Verification items for the finished model (mm, model axes). Face numbers are marked on the shaded views. A direction names the side the tool comes from. Give positions to 0.01 mm unless a question says otherwise; leave off trailing zeros. Order: outer loops, then holes, each group sorted by start corner. A loop starts at its lowest first (then second) coordinate and runs counter-clockwise, first axis right, second up. Notation, with made-up numbers: M 49,24 L 79,24 A16 ccw 79,39 Z; hole C -30.75,65 d8. An arc over 180 degrees is marked long. Answer as a JSON object with one key per item and string values.
Autodesk Inventor part; units mm, degrees
ref_plane "YZ Plane" through (0, 0, 0) normal (1, 0, 0) x (0, 1, 0)
ref_plane "XZ Plane" through (0, 0, 0) normal (0, 1, 0) x (-1, 0, 0)
ref_plane "XY Plane" through (0, 0, 0) normal (0, 0, 1) x (1, 0, 0)
sketch "Sketch1" plane through (0, 0, 0) normal (0, 0, 1) x (1, 0, 0)
  line L0 (3.75, -3.75) -> (-3.75, -3.75) construction
  line L1 (-3.75, -3.75) -> (-3.75, 3.75) construction
  line L2 (-3.75, 3.75) -> (3.75, 3.75) construction
  line L3 (3.75, 3.75) -> (3.75, -3.75) construction
  line L4 (3.75, -3.75) -> (-3.75, 3.75) construction
  line L5 (-3.75, -3.75) -> (3.75, 3.75) construction
  line L6 (-6.9, -3.15) -> (-4.9, -3.15) construction
  line L7 (-4.9, -3.15) -> (-4.9, -1.15) construction
  line L8 (-4.9, -1.15) -> (-6.9, -1.15) construction
  line L9 (-6.9, -1.15) -> (-6.9, -3.15) construction
  line L10 (-6.9, -3.15) -> (-4.9, -1.15) construction
  line L11 (-4.9, -3.15) -> (-6.9, -1.15) construction
  line L12 (-0.5, -8) -> (2.5, -8) construction
  line L13 (2.5, -8) -> (2.5, -5) construction
  line L14 (2.5, -5) -> (-0.5, -5) construction
  line L15 (-0.5, -5) -> (-0.5, -8) construction
  line L16 (-0.5, -8) -> (2.5, -5) construction
  line L17 (2.5, -8) -> (-0.5, -5) construction
  circle A0 centre (-11.1, -2.4) radius 1.1
  circle A1 centre (-11.1, -2.4) radius 2
  circle A2 centre (11.3, 1.7) radius 1.1
  circle A3 centre (11.3, 1.7) radius 2
  line L18 (-2.1716, -8.5) -> (3.9284, -8.5)
  line L19 (3.9284, -8.5) -> (12.7142, 0.2858)
  line L20 (12.7142, 3.1142) -> (11.5784, 4.25)
  line L21 (11.5784, 4.25) -> (-7.2784, 4.25)
  line L22 (-7.2784, 4.25) -> (-12.5142, -0.9858)
  line L23 (-12, -7.9) -> (-9, -7.9) construction
  line L24 (-9, -7.9) -> (-9, -4.9) construction
  line L25 (-9, -4.9) -> (-12, -4.9) construction
  line L26 (-12, -4.9) -> (-12, -7.9) construction
  line L27 (-12, -7.9) -> (-9, -4.9) construction
  line L28 (-9, -7.9) -> (-12, -4.9) construction
  line L29 (-11.1, -4.4) -> (-6.2716, -4.4)
  line L30 (-6.2716, -4.4) -> (-2.1716, -8.5)
  line L31 (-4.25, 4.25) -> (-4.25, -2.65)
  arc A4 (-4.25, -2.65) -> (-2.65, -4.25) centre (-2.65, -2.65) ccw
  line L32 (-2.65, -4.25) -> (2.65, -4.25)
  arc A5 (2.65, -4.25) -> (4.25, -2.65) centre (2.65, -2.65) ccw
  line L33 (4.25, -2.65) -> (4.25, 4.25)
  line L34 (-10.9284, 0.6) -> (-4.25, 0.6)
  line L35 (3, -8.5) -> (3, -5)
  arc A6 (3, -5) -> (2.5, -4.5) centre (2.5, -5) ccw
  line L36 (-1, -8.5) -> (-1, -5)
  line L37 (2.5, -4.5) -> (-0.5, -4.5)
  arc A7 (-0.5, -4.5) -> (-1, -5) centre (-0.5, -5) ccw
  point P0 (0, 0)
  point P1 (-5.9, -2.15)
  point P2 (1, -6.5)
  point P3 (-10.5, -6.4)
  dimension "d0" = 6.5
  dimension "d1" = 1
  dimension "d2" = 5.9
  dimension "d3" = 2.15
  dimension "d4" = 7.5
  dimension "d5" = 3
  dimension "d6" = 2
  dimension "d7" = 2.2
  dimension "d8" = 4
  dimension "d9" = 11.1
  dimension "d10" = 2.4
  dimension "d11" = 11.3
  dimension "d12" = 1.7
  dimension "d16" = 0.5
  dimension "d17" = 0.5
  dimension "d20" = 10.5
  dimension "d21" = 6.4
  dimension "d22" = 3
  dimension "d23" = 135
  dimension "d24" = 1.6
  dimension "d25" = 0.5
  dimension "d28" = 3
extrude "Extrusion1" add sketch "Sketch1" against normal blind 3.9 contours A0 | A1 | A1 L22 L34 L31 A4 L32 A5 L33 L21 L20 A3 L19 L18 L35 A6 L37 A7 L36 L30 L29 | L22 L21 L31 L34 | L31 L21 L33 A5 L32 A4 | L36 A7 L37 A6 L35 L18 | A3 | A2
extrude "Extrusion2" cut sketch "Sketch1" against normal blind 3.4 contours L31 L21 L33 A5 L32 A4
extrude "Extrusion3" cut sketch "Sketch1" against normal blind 1.9 contours L22 L21 L31 L34
extrude "Extrusion4" cut sketch "Sketch1" against normal blind 1.3 contours A1 L22 L34 L31 A4 L32 A5 L33 L21 L20 A3 L19 L18 L35 A6 L37 A7 L36 L30 L29
extrude "Extrusion5" cut sketch "Sketch1" against normal blind 1.185 contours L36 A7 L37 A6 L35 L18
hole "Hole1" at (-11.1, -2.4, 0) at (11.3, 1.7, 0) direction (0, 0, -1) diameter 1.567 end through all
equation "\"d17\" = d16"
properties part number "EPS_RegulatorHeatsink" material "Copper"
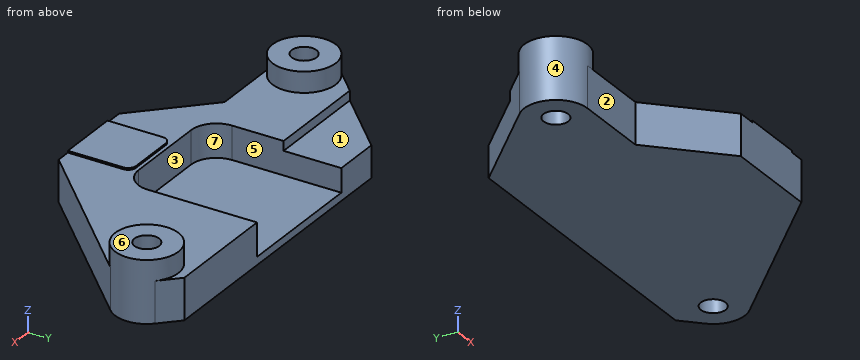
Q1. Release check for a two-part mould opening along X. For the marked faces 4, 5, 6 and 7 record: +X half, -X half, draft (parallel to the pull), parting line (faces both ways), or undercut.
Resolved:
{"face 4": "parting line", "face 5": "undercut", "face 6": "draft", "face 7": "undercut"}
Q2. Section check C-C on y = 1.7. Record the cut outline in (x, z), then the cut area to 3 significant figures.
Resolved:
{"outline": "M -9.83,-3.9 L 10.52,-3.9 L 10.52,0 L 9.3,0 L 9.3,-1.3 L 4.25,-1.3 L 4.25,-3.4 L -4.25,-3.4 L -4.25,-1.9 L -9.83,-1.9 Z; M 12.08,-3.9 L 13.3,-3.9 L 13.3,0 L 12.08,0 Z", "area": "38.0 mm²"}
Q3. Section check B-B on z = -2.25. Record the cut outline in (x, y), then the cut area to 3 significant figures.
Resolved:
{"outline": "M -12.51,-0.99 A2 ccw -11.1,-4.4 L -6.27,-4.4 L -2.17,-8.5 L 3.93,-8.5 L 12.71,0.29 A2 ccw 12.71,3.11 L 11.58,4.25 L 4.25,4.25 L 4.25,-2.65 A1.6 cw 2.65,-4.25 L -2.65,-4.25 A1.6 cw -4.25,-2.65 L -4.25,4.25 L -7.28,4.25 Z; hole C -11.1,-2.4 d1.57; hole C 11.3,1.7 d1.57", "area": "162 mm²"}
Q4. Section check A-A on x = 11.3. Record the cut outline in (y, z), then the cut area to 3 significant figures.
Resolved:
{"outline": "M -1.13,-3.9 L 0.92,-3.9 L 0.92,0 L -0.3,0 L -0.3,-1.3 L -1.13,-1.3 Z; M 2.48,-3.9 L 4.25,-3.9 L 4.25,-1.3 L 3.7,-1.3 L 3.7,0 L 2.48,0 Z", "area": "13.1 mm²"}
Q5. Gauge pin test, flat ends, axial feed: pin 1 Ø3 at (x, y) = (1.5, -6.5) entering from +Z (3 decimals); pin 2 Ø0.5 at (x, z) = (-9, -1.5) entering from +Y; pin 3 Ø2.5 at (x, y) = (2, 0.5) entering from +Z. Record the tip position at first contact, or that the pin passes through.
Resolved:
{"pin 1": "stops at z = -1.185", "pin 2": "stops at y = 0.6", "pin 3": "stops at z = -3.4"}
Q6. Material ranges on L1, parallel to X at y = -2.4, z = -2.3; L2, parallel to X at y = 2, z = -2.65; L3, parallel to Y at x = 11.3, z = -1.25, recorded low to high.
Resolved:
{"L1": "x = -13.1 to -11.88, -10.32 to -4.25, 4.25 to 10.03", "L2": "x = -9.53 to -4.25, 4.25 to 10.58, 12.02 to 13.28", "L3": "y = -0.3 to 0.92, 2.48 to 3.7"}
Q7. Tool access check on the marked faces 1, 2 and 3. Record the directions out of +Z, -Z, +X, -X, +Y, -Y that give a thin tool (end or side, any length) a straight path to the whole face; none if there is none.
Resolved:
{"face 1": "+Z, -X, +Y", "face 2": "+Z, -Z, -X, -Y", "face 3": "+Z, +Y"}
Q8. Section check D-D on y = -1.25. Record the cut outline in (x, z), then the cut area to 3 significant figures.
Resolved:
{"outline": "M -12.74,-3.9 L 11.18,-3.9 L 11.18,-1.3 L 4.25,-1.3 L 4.25,-3.4 L -4.25,-3.4 L -4.25,-1.3 L -9.46,-1.3 L -9.46,0 L -12.74,0 Z", "area": "48.6 mm²"}
